Model file for the job. Use its own axes, mm. Coordinates: 2 decimals unless noted, no trailing zeros. Loops run counter-clockwise (first coordinate to the right, second up) from the corner with the lowest first, then second, coordinate; pieces in that order, holes last. Notation, with made-up numbers: (-11, -6) - (10, -6) arc R22 ccw to (10, 3) - close; hole circle Ø11 at (26.25, 59.25). An arc over 180 degrees is marked (long way). Write each question's results on one line, items separated by ' | '. Start each with the question number.
```python
from build123d import *

# Parameters (mm, degrees)
ESQUISSE1_R          = 7
ESQUISSE1_R_2        = 4
BASE_EXTRUSION_DEPTH = 27.6
CHANFREIN2_SIZE      = 0.5


with BuildPart() as part:
    # Esquisse1 → Base-Extrusion (new body)
    with BuildSketch(Plane.XY):
        with Locations(Location((0, 0, 0), (0, 0, 180))):
            Circle(ESQUISSE1_R)
        with Locations(Location((0, 0, 0), (0, 0, 180))):
            Circle(ESQUISSE1_R_2, mode=Mode.SUBTRACT)
    extrude(amount=BASE_EXTRUSION_DEPTH)

    # Chanfrein2
    chanfrein2_edges = [part.edges().sort_by_distance(p)[0] for p in [
        (7, 0, 0),
        (7, 0, 27.6),
        (4, 0, 0),
        (4, 0, 27.6),
    ]]
    chamfer(chanfrein2_edges, length=CHANFREIN2_SIZE)


solid = part.part
```
Q1. Mould opens along Y. For faces 1 (the flat face through (1.54, -4.42, 27.6)), 2 (the cylindrical face through (0.867, 3.905, 13.614)), 3 (the cylindrical face through (-6.466, 2.681, 13.614)) say: +Y half, -Y half, draft (parallel to the pull), parting line (faces both ways), or undercut.
Q2. Cut at C-C (z = 1.75). List the corners of the cut face in (x, y).
Q3. Pin check, flat tips, straight feed: pin 1 (5 mm diameter, centred on x = 0, y = 0, fed in from +Z); pin 2 (5 mm diameter, centred on x = 1.5, z = 5, fed in from -Y); pin 3 (4 mm diameter, centred on x = -2, y = -0.5, fed in from -Z); pin 4 (2 mm diameter, centred on y = -1.5, z = 7.5, fed in from -X). Stop position of each tip, or through.
Q4. Drill centre lines: L1, parallel to Y at x = 0, z = 16.5; L2, parallel to X at y = -1.5, z = 19.25; L3, parallel to X at y = 1.25, z = 20.5. Where is each one in solid material? Low to high. Write a range as from..to.
Q5. Cut at A-A (x = 0). List the corners of the cut face in (y, z).
Check result:
1) face 1: draft | face 2: undercut | face 3: parting line
2) outline: circle Ø14 at (0, 0); hole circle Ø8 at (0, 0)
3) pin 1: through | pin 2: y = -7 | pin 3: z = 0.44 | pin 4: x = -6.98
4) L1: -7..-4, 4..7 | L2: -6.84..-3.71, 3.71..6.84 | L3: -6.89..-3.8, 3.8..6.89
5) outline: (-7, 0.5) - (-6.5, 0) - (-4.5, 0) - (-4, 0.5) - (-4, 27.1) - (-4.5, 27.6) - (-6.5, 27.6) - (-7, 27.1) - close; (4, 0.5) - (4.5, 0) - (6.5, 0) - (7, 0.5) - (7, 27.1) - (6.5, 27.6) - (4.5, 27.6) - (4, 27.1) - close
